Part model, mm, in its own coordinate system. A direction names the side the tool comes from. Coordinates: 2 decimals unless noted, no trailing zeros. Loops run counter-clockwise (first coordinate to the right, second up) from the corner with the lowest first, then second, coordinate; pieces in that order, holes last.
```python
from build123d import *

# Parameters (mm, degrees)
F0_R     = 17.5
F1_DEPTH = 2
F2_R     = 13.5
F3_DEPTH = 1
F5_SIZE  = 0.5


with BuildPart() as f1:
    # F0 (on Top) → F1 (new body)
    with BuildSketch(Plane.XY):
        Circle(F0_R)
    extrude(amount=F1_DEPTH)

    # F2 (on face) → F3 (cut)
    with BuildSketch(Plane(origin=(0, 0, 0), x_dir=(1, 0, 0), z_dir=(0, 0, -1))):
        Circle(F2_R)
    extrude(amount=-F3_DEPTH, mode=Mode.SUBTRACT)

    # F4: F1 across face


with BuildPart() as f1_1:
    add(f1.part)
    add(f1.part.mirror(Plane.XY.offset(2)))

    # F5
    f5_edges = [f1_1.edges().sort_by_distance(p)[0] for p in [
        (-17.5, 0, 0),
        (17.5, 0, 2),
        (-17.5, 0, 4),
    ]]
    chamfer(f5_edges, length=F5_SIZE)


solid = f1_1.part
```
Q1. Drop flat-ended pins along their axis: P1, Ø2, axis at x = -9.5, z = 0.5, coming from the +Y side; P2, Ø2, axis at x = 4.5, y = 8, coming from the +Z side; P3, Ø13.5, axis at x = -4.5, y = 1.5, coming from the -Z side. Give the stop position or say it passes through.
Q2. Probe line 1 (Y direction, x = 0, z = 3.3); line 2 (Z direction, x = 7, y = 10); line 3 (Y direction, x = -9.5, z = 0.6). List the from-to ranges inside material, lowest first.
Q3. Mould opens along Y. For faces 4 (the flat face through (5, 13, 4)), 5 (the cylindrical face through (-2.93, 13.18, 0.49)) say: released by +Y, released by -Y, zero draft, split by the parting line, or undercut.
Q4. Tool access for faces 1 (the flat face through (5, 13, 0)), 2 (the cylindrical face through (-2.93, 13.18, 3.51)), 3 (the flat face through (0, 0, 1)): list every direction of +Z, -Z, +X, -X, +Y, -Y with a clear straight run to the whole face (end or side of a thin tool).
Q5. Saw through at A-A (x = 0). List the corners of the cut face in (y, z).
Checked values:
1. P1: stops at y = 15.3
1. P2: stops at z = 3
1. P3: stops at z = 1
2. line 1: y = -17.5 to -13.5, 13.5 to 17.5
2. line 2: z = 1 to 3
2. line 3: y = -14.7 to -9.59, 9.59 to 14.7
3. face 4: zero draft
3. face 5: undercut
4. face 1: -Z, +X, -X, +Y, -Y
4. face 2: +Z
4. face 3: -Z
5. outline: (-17.5, 0.5) - (-17, 0) - (-13.5, 0) - (-13.5, 1) - (13.5, 1) - (13.5, 0) - (17, 0) - (17.5, 0.5) - (17.5, 3.5) - (17, 4) - (13.5, 4) - (13.5, 3) - (-13.5, 3) - (-13.5, 4) - (-17, 4) - (-17.5, 3.5) - close
